For this review, take the finished solid that the model builds, in its own axes (mm). Face numbers are marked on the shaded views. A direction names the side the tool comes from. Coordinates: 2 decimals unless noted, no trailing zeros. Order: outer loops, then holes, each group sorted by start corner. A loop starts at its lowest first (then second) coordinate and runs counter-clockwise, first axis right, second up.
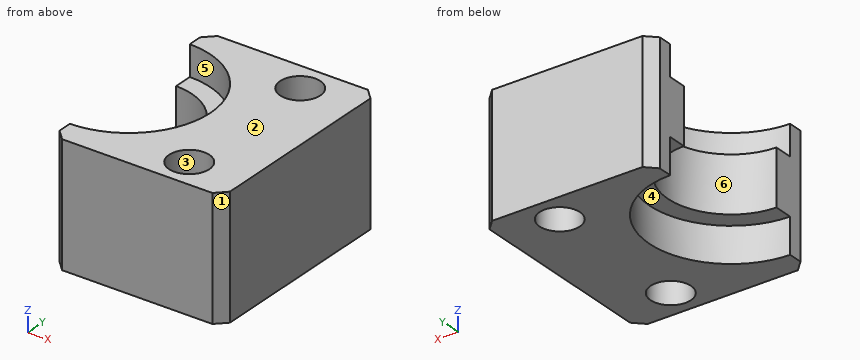
from build123d import *

# Parameters (mm, degrees)
F0_R     = 2
F1_DEPTH = 12
F2_R     = 8.1
F3_DEPTH = 3
F4_R     = 6.25
F5_DEPTH = 5.5
F6_R     = 8.1
F7_DEPTH = 25
F8_SIZE  = 1


with BuildPart() as f1:
    # F0 (on Top) → F1 (new body)
    with BuildSketch(Plane.XY):
        with BuildLine():
            Line((-0.9, -10.5), (16, -10.5))
            Line((16, -10.5), (16, 10.5))
            Line((16, 10.5), (-0.9, 10.5))
            Line((-0.9, 10.5), (-0.9, 0.9949874371))
            ThreePointArc((-0.9, 0.9949874371), (0, 0), (-0.9, -0.9949874371))
            Line((-0.9, -0.9949874371), (-0.9, -10.5))
        make_face()
        with Locations((10.5, -7.5)):
            Circle(F0_R, mode=Mode.SUBTRACT)
        with Locations((10.5, 7.5)):
            Circle(F0_R, mode=Mode.SUBTRACT)
    extrude(amount=F1_DEPTH)

    # F2 (on face) → F3 (cut)
    with BuildSketch(Plane.XY.offset(12)):
        with Locations((-1, 0)):
            Circle(F2_R)
    extrude(amount=-F3_DEPTH, mode=Mode.SUBTRACT)

    # F4 (on face) → F5 (cut)
    with BuildSketch(Plane.XY.offset(9)):
        with Locations((-1, 0)):
            Circle(F4_R)
    extrude(amount=-F5_DEPTH, mode=Mode.SUBTRACT)

    # F6 (on face) → F7 (cut)
    with BuildSketch(Plane.XY.offset(3.5)):
        with Locations((-1, 0)):
            Circle(F6_R)
    extrude(amount=-F7_DEPTH, mode=Mode.SUBTRACT)

    # F8
    f8_edges = [f1.edges().sort_by_distance(p)[0] for p in [
        (16, 10.5, 6),
        (16, -10.5, 6),
        (-0.9, -10.5, 6),
        (-0.9, 10.5, 6),
    ]]
    chamfer(f8_edges, length=F8_SIZE)


solid = f1.part
1. Take a section at C-C, the plane x = 1.25. Give the boundary of the cut face in (y, z).
Answer below:
outline: (-10.5, 0) - (-7.78, 0) - (-7.78, 3.5) - (-5.83, 3.5) - (-5.83, 9) - (-7.78, 9) - (-7.78, 12) - (-10.5, 12) - close; (5.83, 3.5) - (7.78, 3.5) - (7.78, 0) - (10.5, 0) - (10.5, 12) - (7.78, 12) - (7.78, 9) - (5.83, 9) - close
2. Take a section at A-A, the plane x = 10.5. Give the boundary of the cut face in (y, z).
Answer below:
outline: (-10.5, 0) - (-9.5, 0) - (-9.5, 12) - (-10.5, 12) - close; (-5.5, 0) - (5.5, 0) - (5.5, 12) - (-5.5, 12) - close; (9.5, 0) - (10.5, 0) - (10.5, 12) - (9.5, 12) - close
3. Take a section at D-D, the plane y = -7. Give the boundary of the cut face in (x, z), plus the area to 3 significant figures.
Answer below:
outline: (-0.9, 3.5) - (3.08, 3.5) - (3.08, 0) - (8.56, 0) - (8.56, 12) - (3.08, 12) - (3.08, 9) - (-0.9, 9) - close; (12.44, 0) - (16, 0) - (16, 12) - (12.44, 12) - close
area: 130 mm2
4. Machinability: for the marked faces 4, 5 and 6, which of the approach directions +Z, -Z, +X, -X, +Y, -Y give a long, thin tool a straight path to every point of the face, cutting with its end or side? Answer none if there is none.
Answer below:
face 4: -Z, -X
face 5: +Z, -X
face 6: +Z, -Z, -X
5. Take a section at B-B, the plane z = 11. Give the boundary of the cut face in (x, y), plus the area to 3 significant figures.
Answer below:
outline: (-0.9, -9.5) - (0.1, -10.5) - (15, -10.5) - (16, -9.5) - (16, 9.5) - (15, 10.5) - (0.1, 10.5) - (-0.9, 9.5) - (-0.9, 8.1) arc R8.1 cw to (-0.9, -8.1) - close; hole circle Ø4 at (10.5, -7.5); hole circle Ø4 at (10.5, 7.5)
area: 226 mm2
6. The part is to be moulded in two halves that separate along Y. For the marked faces 1, 2 and 3, say which applies: +Y half, -Y half, draft (parallel to the pull), parting line (faces both ways), or undercut.
Answer below:
face 1: -Y half
face 2: draft
face 3: undercut
7. To check wall thickness, follow L1, parallel to Y at x = 10.5, z = 5.75; L2, parallel to Y at x = 8.75, z = 9; L3, parallel to X at y = -0.25, z = 1.25. State the ranges of each line that lie inside material, in increasing order.
Answer below:
L1: y = -10.5 to -9.5, -5.5 to 5.5, 9.5 to 10.5
L2: y = -10.5 to -8.47, -6.53 to 6.53, 8.47 to 10.5
L3: x = 7.1 to 16
